Read the model definition and answer for the solid it produces. Units are mm, in the model's axes. Coordinates: 2 decimals unless noted, no trailing zeros. Write each loop counter-clockwise with the first axis right and the second up, starting at its lowest first coordinate (ties: lowest second). Pieces come first, ordered by that corner, then holes. Notation, with made-up numbers: (74, 17.5) -> (123, 17.5) arc R33 ccw to (123, 51.5) -> close; hole circle Ø3 at (49, 87.25). An arc over 180 degrees is marked (long way). Answer in a Markdown table with one row per item. Add a question column.
Item 1: Straight lines are drawn through the part: line 1 (Z direction, x = 3.25, y = 3.05) (3 decimals); line 2 (Z direction, x = 1.75, y = 3.15) (3 decimals); line 3 (X direction, y = 3.2, z = 146.8). For each, find the intervals that lie inside material, in ascending order. Write a range as from..to.
Item 2: Given pin 1 Ø1 at (x, y) = (3, 3) entering from -Z; pin 2 Ø0.8 at (y, z) = (3.5, 164.5) entering from +X; pin 3 Ø1 at (y, z) = (1, 64.5) entering from -X, each flat-ended and moving along its own axis, determine where each tip first touches the part or whether it passes through.
Item 3: Section A-A on z = 57 is taken. Write down the section's boundary in (x, y).
Item 4: Section B-B on y = 1.25 is taken. Write down the section's boundary in (x, z).
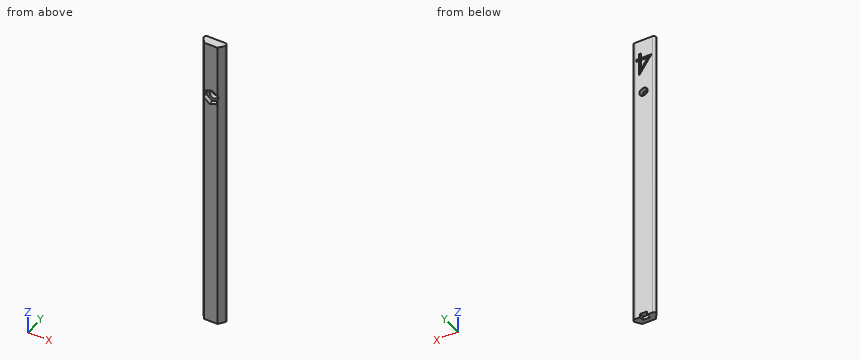
```python
from build123d import *

# Parameters (mm, degrees)
BOSS_EXTRUDE1_DEPTH = 171.2
FILLET1_R           = 1
SKETCH2_R           = 1.8
CUT_EXTRUDE1_DEPTH  = 200
CUT_EXTRUDE2_DEPTH  = 2
LPATTERN1_COUNT     = 3
LPATTERN1_PITCH     = 116
CUT_EXTRUDE3_DEPTH  = 1
THICKEN1_T1         = 40
SKETCH5_W           = 43.187551832
SKETCH5_H           = 200
CUT_EXTRUDE4_DEPTH  = 10
SKETCH7_W           = 3
SKETCH7_H           = 3
CUT_EXTRUDE5_DEPTH  = 2


with BuildPart() as part:
    # Sketch1 → Boss-Extrude1 (new body)
    with BuildSketch(Plane.XY):
        Polygon((0, 0), (5.8, 0), (8.7, 3.9), (-2.9, 3.9), align=None)
    extrude(amount=BOSS_EXTRUDE1_DEPTH)

    # Fillet1
    fillet1_edges = [part.edges().sort_by_distance(p)[0] for p in [
        (-2.9, 3.9, 85.6),
        (8.7, 3.9, 85.6),
    ]]
    fillet(fillet1_edges, radius=FILLET1_R)

    # Sketch2 → Cut-Extrude1 (cut)
    with BuildSketch(Plane.XZ):
        with Locations(Location((2.9, 146.8, 0), (0, 0, 270))):
            Circle(SKETCH2_R)
    cut_extrude1 = extrude(amount=-CUT_EXTRUDE1_DEPTH, mode=Mode.SUBTRACT)

    # Sketch3 → Cut-Extrude2 (cut)
    with BuildSketch(Plane.XZ):
        Polygon((3.536306697, 150.087620282), (0.370990666, 148.994867905), (-0.265316031, 145.707247623), (2.263693303, 143.512379718), (5.429009334, 144.605132095), (6.065316031, 147.892752377), align=None)
    cut_extrude2 = extrude(amount=-CUT_EXTRUDE2_DEPTH, mode=Mode.SUBTRACT)

    # LPattern1: Cut-Extrude1, Cut-Extrude2 ×3
    with Locations(*[(0, 0, -i * LPATTERN1_PITCH) for i in range(1, LPATTERN1_COUNT)]):
        add(cut_extrude1, mode=Mode.SUBTRACT)
        add(cut_extrude2, mode=Mode.SUBTRACT)

    # Sketch4 → Cut-Extrude3 (cut)
    with BuildSketch(Plane(origin=(0, 3.9, 0), x_dir=(1, 0, 0), z_dir=(0, 1, 0))):
        Polygon((4.655544406, -155.430769231), (4.829177218, -155.430769231), (4.829177218, -162.025), (5.92821568, -162.025), (5.92821568, -163.001923077), (4.829177218, -163.001923077), (4.829177218, -165.2), (3.974369526, -165.2), (3.974369526, -163.001923077), (-0.543899705, -163.001923077), align=None)
        Polygon((3.974369526, -162.025), (3.974369526, -157.888341346), (1.135186834, -162.025), align=None, mode=Mode.SUBTRACT)
    extrude(amount=-CUT_EXTRUDE3_DEPTH, mode=Mode.SUBTRACT)

    # Surface-Offset1: a surface, a copy of 1 face of the part
    surface_offset1_1 = part.part.faces().sort_by_distance((2.9, 2.093393293, 0))[0]
    add(Solid.thicken(surface_offset1_1, THICKEN1_T1))

    # Sketch5 → Cut-Extrude4 (cut)
    with BuildSketch(Plane(origin=(0, 3.9, 0), x_dir=(1, 0, 0), z_dir=(0, 1, 0))):
        with Locations((8.67861609, 58.2)):
            Rectangle(SKETCH5_W, SKETCH5_H)
    extrude(amount=-CUT_EXTRUDE4_DEPTH, mode=Mode.SUBTRACT)

    # Sketch7 → Cut-Extrude5 (cut)
    with BuildSketch(Plane(origin=(0, 3.9, 0), x_dir=(1, 0, 0), z_dir=(0, 1, 0))):
        with Locations((2.9, -41.8)):
            Rectangle(SKETCH7_W, SKETCH7_H)
    extrude(amount=-CUT_EXTRUDE5_DEPTH, mode=Mode.SUBTRACT)


solid = part.part
```
Results below:
| question | item | result |
|---|---|---|
| 1 | line 1 | z = 43.3..145.034, 148.566..157.477, 158.944..162.025, 163.002..171.2 |
| 1 | line 2 | z = 43.3..145.415, 148.185..159.662, 161.129..162.025, 163.002..171.2 |
| 1 | line 3 | x = -1.86..1.1, 4.7..7.66 |
| 2 | pin 1 | stops at z = 43.3 |
| 2 | pin 2 | stops at x = 7.69 |
| 2 | pin 3 | stops at x = -1.12 |
| 3 | outline | (-1.71, 2.3) -> (0, 0) -> (5.8, 0) -> (7.51, 2.3) arc R1 ccw to (6.71, 3.9) -> (-0.91, 3.9) arc R1 ccw to start |
| 4 | outline | (-0.93, 41.8) -> (6.73, 41.8) -> (6.73, 171.2) -> (-0.93, 171.2) -> close; hole (-0.27, 145.71) -> (2.26, 143.51) -> (5.43, 144.61) -> (6.07, 147.89) -> (3.54, 150.09) -> (0.37, 148.99) -> close |
